from build123d import *

# Parameters (mm, degrees)
F0_R     = 13.95
F1_DEPTH = 7
F2_R     = 11
F3_DEPTH = 4
F4_R     = 7.75
F5_DEPTH = 25
F6_W     = 2.5
F6_H     = 2.5
F8_W     = 5
F8_H     = 9
F9_DEPTH = 25


with BuildPart() as f1:
    # F0 (on Top) → F1 (new body)
    with BuildSketch(Plane.XY):
        Circle(F0_R)
    extrude(amount=F1_DEPTH)

    # F2 (on face) → F3 (cut)
    with BuildSketch(Plane(origin=(0, 0, 0), x_dir=(1, 0, 0), z_dir=(0, 0, -1))):
        with Locations((0, -0.393073)):
            Circle(F2_R)
    extrude(amount=-F3_DEPTH, mode=Mode.SUBTRACT)

    # F4 (on face) → F5 (cut)
    with BuildSketch(Plane(origin=(0, 0, 4), x_dir=(1, 0, 0), z_dir=(0, 0, -1))):
        Circle(F4_R)
    extrude(amount=-F5_DEPTH, mode=Mode.SUBTRACT)

    # F6 (on Front) → F7 (revolve)
    with BuildSketch(Plane.XZ):
        with Locations((15.190209, 1.25)):
            Rectangle(F6_W, F6_H)
    revolve(axis=Axis((0, 0, 5.198275), (0, 0, 1)))

    # F8 (on Top) → F9 (cut)
    with BuildSketch(Plane.XY):
        with Locations((0, 4.5)):
            Rectangle(F8_W, F8_H)
    extrude(amount=F9_DEPTH, mode=Mode.SUBTRACT)


solid = f1.part
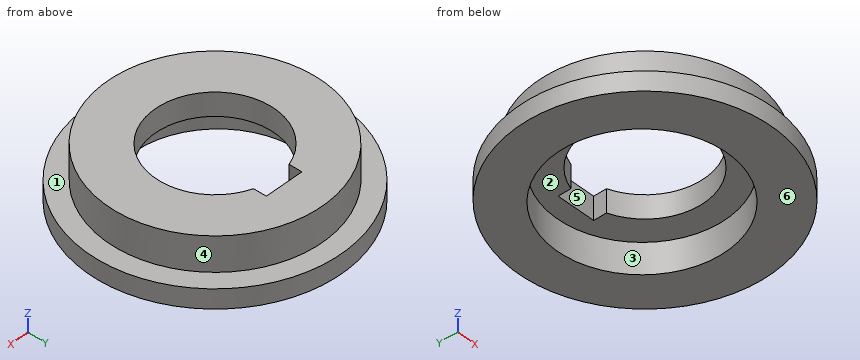
The model under review builds one solid part; all positions refer to its coordinate system, in mm. Face numbers are marked on the shaded views. A direction names the side the tool comes from. Give positions to 0.01 mm unless a question says otherwise; leave off trailing zeros. Write each loop counter-clockwise with the first axis right and the second up, starting at its lowest first coordinate (ties: lowest second). Pieces come first, ordered by that corner, then holes.
1. For P1, Ø17.5, axis at x = 0, y = 0.39, coming from the +Z side; P2, Ø0.5, axis at y = 8, z = 5, coming from the +X side; P3, Ø2.5, axis at x = -0.5, z = 6, coming from the -Y side; P4, Ø1.3, axis at y = 8, z = 5.5, coming from the -X side, all flat-tipped, find the tip position at first contact; note any pin that passes through.
2. Add section B-B, the plane y = -2. Write out the cut boundary in (x, z), plus the area to 3 significant figures.
3. Add section C-C, the plane z = 5.5. Write out the cut boundary in (x, y), plus the area to 3 significant figures.
4. Draft analysis for pull direction X (two halves, no side actions). For the marked faces 1, 2, 3 and 4, state which applies: +X half, -X half, draft (parallel to the pull), parting line (faces both ways), or undercut.
5. Tool access review of the marked faces 5 and 6: name each direction out of +Z, -Z, +X, -X, +Y, -Y from which nothing blocks a thin tool from reaching the whole face with its end or side.
6. Add section D-D, the plane x = -13. Write out the cut boundary in (y, z), plus the area to 3 significant figures.
7. Add section A-A, the plane x = 0. Write out the cut boundary in (y, z), plus the area to 3 significant figures.
8. Wall thickness on L1, parallel to Y at x = 0, z = 3.25; L2, parallel to X at y = 0, z = 6.2; L3, parallel to Y at x = 0, z = 1: over which ranges is each line inside the solid? List them lowest first.
Worked answers:
1. P1: stops at z = 7
1. P2: stops at x = 11.6
1. P3: stops at y = -13.95
1. P4: stops at x = -11.86
2. outline: (-16.32, 0) - (-10.74, 0) - (-10.74, 4) - (-7.49, 4) - (-7.49, 7) - (-13.81, 7) - (-13.81, 2.5) - (-16.32, 2.5) - close; (7.49, 4) - (10.74, 4) - (10.74, 0) - (16.32, 0) - (16.32, 2.5) - (13.81, 2.5) - (13.81, 7) - (7.49, 7) - close
2. area: 75.0 mm2
3. outline: circle Ø27.9 at (0, 0); hole (-2.5, 7.34) arc R7.75 ccw (long way) to (2.5, 7.34) - (2.5, 9) - (-2.5, 9) - close
3. area: 416 mm2
4. face 1: draft
4. face 2: undercut
4. face 3: undercut
4. face 4: parting line
5. face 5: +Z, -Z
5. face 6: -Z, +X, -X, +Y, -Y
6. outline: (-10.06, 0) - (10.06, 0) - (10.06, 2.5) - (5.06, 2.5) - (5.06, 7) - (-5.06, 7) - (-5.06, 2.5) - (-10.06, 2.5) - close
6. area: 95.9 mm2
7. outline: (-16.44, 0) - (-10.61, 0) - (-10.61, 4) - (-7.75, 4) - (-7.75, 7) - (-13.95, 7) - (-13.95, 2.5) - (-16.44, 2.5) - close; (9, 4) - (11.39, 4) - (11.39, 0) - (16.44, 0) - (16.44, 2.5) - (13.95, 2.5) - (13.95, 7) - (9, 7) - close
7. area: 69.5 mm2
8. L1: y = -13.95 to -10.61, 11.39 to 13.95
8. L2: x = -13.95 to -7.75, 7.75 to 13.95
8. L3: y = -16.44 to -10.61, 11.39 to 16.44
